from build123d import *

# Parameters (mm, degrees)
SKETCH1_W           = 1208
SKETCH1_H           = 440
BOSS_EXTRUDE1_DEPTH = 4
CUT_EXTRUDE1_DEPTH  = 10
SKETCH3_W           = 1120
SKETCH3_H           = 180
CUT_EXTRUDE2_DEPTH  = 2
SKETCH4_W           = 1100
SKETCH4_H           = 170
CUT_EXTRUDE3_DEPTH  = 3
SKETCH5_R           = 1
CUT_EXTRUDE4_DEPTH  = 1


with BuildPart() as part:
    # Sketch1 → Boss-Extrude1 (new body)
    with BuildSketch(Plane.XY):
        Rectangle(SKETCH1_W, SKETCH1_H)
    extrude(amount=BOSS_EXTRUDE1_DEPTH)

    # Sketch2 → Cut-Extrude1 (cut)
    with BuildSketch(Plane.XY.offset(4)):
        with BuildLine():
            Line((-350, 210), (350, 210))
            ThreePointArc((350, 210), (365, 195), (350, 180))
            Line((350, 180), (-350, 180))
            ThreePointArc((-350, 180), (-365, 195), (-350, 210))
        make_face()
    extrude(amount=-CUT_EXTRUDE1_DEPTH, mode=Mode.SUBTRACT)

    # Sketch3 → Cut-Extrude2 (cut)
    with BuildSketch(Plane.XY.offset(4)):
        with Locations((0, 85)):
            Rectangle(SKETCH3_W, SKETCH3_H)
    extrude(amount=-CUT_EXTRUDE2_DEPTH, mode=Mode.SUBTRACT)

    # Sketch4 → Cut-Extrude3 (cut, through all)
    with BuildSketch(Plane.XY.offset(2)):
        with Locations((0, 85)):
            Rectangle(SKETCH4_W, SKETCH4_H)
    extrude(amount=-CUT_EXTRUDE3_DEPTH, mode=Mode.SUBTRACT)

    # Sketch5 → Cut-Extrude4 (cut)
    with BuildSketch(Plane.XY.offset(2)):
        with Locations((-555, 85)):
            Circle(SKETCH5_R)
    cut_extrude4 = extrude(amount=-CUT_EXTRUDE4_DEPTH, mode=Mode.SUBTRACT)

    # Mirror1: Cut-Extrude4 across plane
    add(cut_extrude4.mirror(Plane(origin=(0, 0, 0), x_dir=(0, 0, 1), z_dir=(1, 0, 0))), mode=Mode.SUBTRACT)


solid = part.part
Can you work these out from the model? Positions are in its coordinate system, mm. Give positions to 0.01 mm unless a question says otherwise; leave off trailing zeros. Order: outer loops, then holes, each group sorted by start corner. A loop starts at its lowest first (then second) coordinate and runs counter-clockwise, first axis right, second up. Notation, with made-up numbers: M 40.25,-23.5 L 44.25,-23.5 A18 cw 44.25,-4.5 Z; hole C 38.5,-0.5 d5. An arc over 180 degrees is marked long. One line per question, with ' | ' between items.
Item 1: Suppose I cut it at A-A, the plane x = -199. Write out the boundary of the cut face in (y, z).
Answer block:
outline: M -220,0 L 0,0 L 0,2 L -5,2 L -5,4 L -220,4 Z; M 170,0 L 180,0 L 180,4 L 175,4 L 175,2 L 170,2 Z; M 210,0 L 220,0 L 220,4 L 210,4 Z
Item 2: Suppose I cut it at D-D, the plane x = 502. Write out the boundary of the cut face in (y, z), then the cut area to 3 significant figures.
Answer block:
outline: M -220,0 L 0,0 L 0,2 L -5,2 L -5,4 L -220,4 Z; M 170,0 L 220,0 L 220,4 L 175,4 L 175,2 L 170,2 Z | area: 1,060 mm2
Item 3: Suppose I cut it at C-C, the plane y = 195. Write out the boundary of the cut face in (x, z).
Answer block:
outline: M -604,0 L -365,0 L -365,4 L -604,4 Z; M 365,0 L 604,0 L 604,4 L 365,4 Z
Item 4: Suppose I cut it at B-B, the plane z = 3.2. Write out the boundary of the cut face in (x, y).
Answer block:
outline: M -604,-220 L 604,-220 L 604,220 L -604,220 Z; hole M -560,-5 L 560,-5 L 560,175 L -560,175 Z; hole M -350,180 L 350,180 A15 ccw 350,210 L -350,210 A15 ccw Z
Item 5: We'd pull the mould along Y, two halves only. Please class faces 1 (the face through (-8, -95, 4)), 2 (the face through (-3, 172, 2)): released by +Y, released by -Y, zero draft, split by the parting line, or undercut.
Answer block:
face 1: zero draft | face 2: undercut
Item 6: Please list where these lines run through material, in increasing order: L1, parallel to Y at x = -180.5, z = 2.75; L2, parallel to Y at x = 135, z = 1.05; L3, parallel to X at y = 195, z = 1.2.
Answer block:
L1: y = -220 to -5, 175 to 180, 210 to 220 | L2: y = -220 to 0, 170 to 180, 210 to 220 | L3: x = -604 to -365, 365 to 604
Item 7: I'm going to push a flat-ended pin straight in: pin 1 Ø0.6 at (x, y) = (555, 85) entering from +Z. Where does the tip first touch, or does it pass through?
Answer block:
pin 1: stops at z = 1
